from build123d import *

# Parameters (mm, degrees)
F1_DEPTH = 53.975
F3_DEPTH = 76.2
F4_R     = 19.05
F5_DEPTH = 63.5
F6_R     = 12.7
F7_R     = 12.7


with BuildPart() as f1:
    # F0 (on Top) → F1 (new body)
    with BuildSketch(Plane.XY):
        Polygon((0, 152.4), (0, 0), (127, 0), (127, 41.275), (152.4, 41.275), (177.8, 152.4), align=None)
    extrude(amount=F1_DEPTH)

    # F2 (on face) → F3 (join)
    with BuildSketch(Plane.XY.offset(53.975)):
        with BuildLine():
            Line((63.5, 100.2127209187), (63.5, 106.5627209187))
            ThreePointArc((63.5, 106.5627209187), (45.5394877579, 99.1232331608), (38.1, 81.1627209187))
            Line((38.1, 81.1627209187), (44.45, 81.1627209187))
            ThreePointArc((44.45, 81.1627209187), (50.0296158184, 94.6331051003), (63.5, 100.2127209187))
        make_face()
        with BuildLine():
            ThreePointArc((88.9, 81.1627209187), (81.4605122421, 99.1232331608), (63.5, 106.5627209187))
            Line((63.5, 106.5627209187), (63.5, 100.2127209187))
            ThreePointArc((63.5, 100.2127209187), (76.9703841816, 94.6331051003), (82.55, 81.1627209187))
            ThreePointArc((82.55, 81.1627209187), (63.5, 62.1127209187), (44.45, 81.1627209187))
            Line((44.45, 81.1627209187), (38.1, 81.1627209187))
            ThreePointArc((38.1, 81.1627209187), (63.5, 55.7627209187), (88.9, 81.1627209187))
        make_face()
        with BuildLine():
            ThreePointArc((82.55, 81.1627209187), (76.9703841816, 94.6331051003), (63.5, 100.2127209187))
            Line((63.5, 100.2127209187), (63.5, 81.1627209187))
            Line((63.5, 81.1627209187), (44.45, 81.1627209187))
            ThreePointArc((44.45, 81.1627209187), (63.5, 62.1127209187), (82.55, 81.1627209187))
        make_face()
        with BuildLine():
            Line((63.5, 81.1627209187), (63.5, 100.2127209187))
            ThreePointArc((63.5, 100.2127209187), (50.0296158184, 94.6331051003), (44.45, 81.1627209187))
            Line((44.45, 81.1627209187), (63.5, 81.1627209187))
        make_face()
    extrude(amount=F3_DEPTH)

    # F4 (on face) → F5 (cut)
    with BuildSketch(Plane.XY.offset(130.175)):
        with Locations((63.5, 81.1627209187)):
            Circle(F4_R)
    extrude(amount=-F5_DEPTH, mode=Mode.SUBTRACT)

    # F6
    f6_edges = [f1.edges().sort_by_distance(p)[0] for p in [
        (88.9, 81.162721, 53.975),
        (127, 20.6375, 53.975),
        (63.5, 0, 53.975),
    ]]
    fillet(f6_edges, radius=F6_R)

    # F7
    f7_edges = [f1.edges().sort_by_distance(p)[0] for p in [
        (0, 82.55, 53.975),
    ]]
    fillet(f7_edges, radius=F7_R)


solid = f1.part
The model under review builds one solid part; all positions refer to its coordinate system, in mm. A direction names the side the tool comes from. Round coordinates to 2 decimals unless told otherwise and drop trailing zeros. Write each loop counter-clockwise with the first axis right and the second up, starting at its lowest first coordinate (ties: lowest second). Pieces come first, ordered by that corner, then holes. Notation, with made-up numbers: M -0.75,18 L 6.25,18 A21 ccw 6.25,42 Z; hole C 66.5,26 d6. An arc over 180 degrees is marked long. Use a Markdown table: item, result. Add a question column.
Q1. The part is to be moulded in two halves that separate along Y. For faces 4 (the face through (70.65, 3.622, 50.156)), 5 (the face through (90, 152.4, 27)), 6 (the face through (123.181, 20.926, 50.353)), 7 (the face through (59.37, 62.566, 98.87)), say which applies: pulls with the +Y half, pulls with the -Y half, needs draft (parallel to the pull), parting line crosses it, or undercut.
Q2. We need section A-A, the plane z = 15.5. State the section outline as (x, y) points (3 decimals).
Q3. To check wall thickness, follow line 1 (Y direction, x = 63, z = 100); line 2 (Y direction, x = 142, z = 33.5) (3 decimals); line 3 (Z direction, x = 146, y = 115) (3 decimals). State the ranges of each line that lie inside material, in increasing order.
Q4. We need section C-C, the plane x = 111.5. State the section outline as (y, z) points (3 decimals).
Q5. Insertion check: pin 1 (8 mm diameter, centred on x = 31.5, y = 56, fed in from +Z); pin 2 (6 mm diameter, centred on y = 61, z = 48, fed in from -X); pin 3 (3 mm diameter, centred on y = 85, z = 52.5, fed in from +X). Each pin has a flat end and moves straight along its axis. Give the tip position at first contact, or say it passes through.
Q6. We need section B-B, the plane y = 20.5. State the section outline as (x, z) points (3 decimals).
Q7. We need section D-D, the plane z = 76. State the section outline as (x, y) points.
Q8. Machinability: for faces 1 (the face through (63, 81, 66.675)), 2 (the face through (69, 0, 20)), 3 (the face through (127, 20, 20)), which of the approach directions +Z, -Z, +X, -X, +Y, -Y give a long, thin tool a straight path to every point of the face, cutting with its end or side? Answer none if there is none.
Findings below:
| question | item | result |
|---|---|---|
| 1 | face 4 | pulls with the -Y half |
| 1 | face 5 | pulls with the +Y half |
| 1 | face 6 | needs draft |
| 1 | face 7 | undercut |
| 2 | outline | M 0,12.7 A12.7 ccw 12.7,0 L 127,0 L 127,41.275 L 152.4,41.275 L 177.8,152.4 L 0,152.4 Z |
| 3 | line 1 | y = 55.77 to 62.12, 100.21 to 106.56 |
| 3 | line 2 | y = 41.275 to 152.4 |
| 3 | line 3 | z = 0 to 53.975 |
| 4 | outline | M 0,0 L 152.4,0 L 152.4,53.975 L 12.7,53.975 A12.7 ccw 0,41.275 Z |
| 5 | pin 1 | stops at z = 54.05 |
| 5 | pin 2 | stops at x = 0.56 |
| 5 | pin 3 | stops at x = 162.74 |
| 6 | outline | M 0,0 L 127,0 L 127,41.275 A12.7 ccw 114.3,53.975 L 12.7,53.975 A12.7 ccw 0,41.275 Z |
| 7 | outline | C 63.5,81.16 d50.8; hole C 63.5,81.16 d38.1 |
| 8 | face 1 | +Z |
| 8 | face 2 | +Z, -Z, +X, -X, -Y |
| 8 | face 3 | +Z, -Z, +X, -Y |
